```python
from build123d import *

# Parameters (mm, degrees)
SKETCH2_R           = 1.5
BOSS_EXTRUDE1_DEPTH = 2.5
SKETCH3_OUTSIDE_W   = 22.086
SKETCH3_OUTSIDE_H   = 21.158
SKETCH3_OUTSIDE_R   = 3
CUT_EXTRUDE1_DEPTH  = 3.25
CUT_EXTRUDE1_DRAFT  = 60
SKETCH4_OUTSIDE_W   = 22.086
SKETCH4_OUTSIDE_H   = 21.158
SKETCH4_OUTSIDE_R   = 3
CUT_EXTRUDE2_DEPTH  = 3.25
CUT_EXTRUDE2_DRAFT  = -60
CHAMFER1_SIZE       = 0.075


with BuildPart() as part:
    # Sketch2 → Boss-Extrude1 (new body)
    with BuildSketch(Plane(origin=(0, 0, 0), x_dir=(1, 0, 0), z_dir=(0, 1, 0))):
        Polygon((3.464101615, 0), (1.732050808, 3), (-1.732050808, 3), (-3.464101615, 0), (-1.732050808, -3), (1.732050808, -3), align=None)
        with Locations(Location((0, 0, 0), (0, 0, 270))):
            Circle(SKETCH2_R, mode=Mode.SUBTRACT)
    extrude(amount=BOSS_EXTRUDE1_DEPTH)


with BuildPart() as cut_extrude1_tool:
    # Sketch3 outside → Cut-Extrude1 (with draft: the straight prism first)
    with BuildSketch(Plane(origin=(0, 0, 0), x_dir=(1, 0, 0), z_dir=(0, 1, 0))):
        Rectangle(SKETCH3_OUTSIDE_W, SKETCH3_OUTSIDE_H)
        Circle(SKETCH3_OUTSIDE_R, mode=Mode.SUBTRACT)
    extrude(amount=CUT_EXTRUDE1_DEPTH)
    # Cut-Extrude1: the draft: its side faces are tilted about the plane it starts from
    cut_extrude1_sides = [cut_extrude1_tool.faces().sort_by_distance(p)[0] for p in [
        (0, 1.625, 10.579),
        (11.043, 1.625, 0),
        (0, 1.625, -10.579),
        (-11.043, 1.625, 0),
        (-3, 1.625, 0),
    ]]
    draft(cut_extrude1_sides, Plane(origin=(0, 0, 0), x_dir=(1, 0, 0), z_dir=(0, 1, 0)), CUT_EXTRUDE1_DRAFT)


with BuildPart() as part_1:
    add(part.part)

    # Cut-Extrude1: cut by cut_extrude1_tool
    add(cut_extrude1_tool.part, mode=Mode.SUBTRACT)


with BuildPart() as cut_extrude2_tool:
    # Sketch4 outside → Cut-Extrude2 (with draft: the straight prism first)
    with BuildSketch(Plane(origin=(0, 2.5, 0), x_dir=(1, 0, 0), z_dir=(0, 1, 0))):
        Rectangle(SKETCH4_OUTSIDE_W, SKETCH4_OUTSIDE_H)
        Circle(SKETCH4_OUTSIDE_R, mode=Mode.SUBTRACT)
    extrude(amount=-CUT_EXTRUDE2_DEPTH)
    # Cut-Extrude2: the draft: its side faces are tilted about the plane it starts from
    cut_extrude2_sides = [cut_extrude2_tool.faces().sort_by_distance(p)[0] for p in [
        (0, 0.875, 10.579),
        (11.043, 0.875, 0),
        (0, 0.875, -10.579),
        (-11.043, 0.875, 0),
        (-3, 0.875, 0),
    ]]
    draft(cut_extrude2_sides, Plane(origin=(0, 2.5, 0), x_dir=(1, 0, 0), z_dir=(0, 1, 0)), CUT_EXTRUDE2_DRAFT)


with BuildPart() as part_2:
    add(part_1.part)

    # Cut-Extrude2: cut by cut_extrude2_tool
    add(cut_extrude2_tool.part, mode=Mode.SUBTRACT)

    # Chamfer1
    chamfer1_edges = [part_2.edges().sort_by_distance(p)[0] for p in [
        (0, 0, -1.5),
        (0, 2.5, -1.5),
    ]]
    chamfer(chamfer1_edges, length=CHAMFER1_SIZE)


solid = part_2.part
```
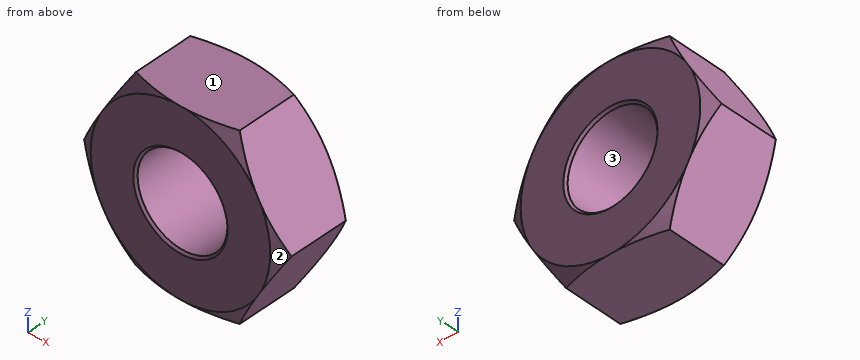
Work out the finished part from the listing and answer in its coordinate system (mm). Face numbers are marked on the shaded views. Give positions to 0.01 mm unless a question says otherwise; leave off trailing zeros. Write each loop counter-clockwise with the first axis right and the second up, starting at its lowest first coordinate (ties: lowest second). Pieces come first, ordered by that corner, then holes. Notation, with made-up numbers: (-12, -14.5) - (-1, -14.5) arc R7 ccw to (-1, -2.5) - close; hole circle Ø4 at (69, -2). An arc over 180 degrees is marked (long way). Use one line per item in the form item = value.
1. Determine the mould class of the marked faces 1, 2 and 3 for opening direction Z: released by +Z, released by -Z, zero draft, split by the parting line, or undercut.
Filled in:
face_1 = released by +Z
face_2 = split by the parting line
face_3 = undercut
2. A cutting plane is placed at A-A (y = 1.5). Write down the section's boundary in (x, z), and give its area (3 significant figures).
Filled in:
outline = (-3.46, 0) - (-1.73, -3) - (1.73, -3) - (3.46, 0) - (1.73, 3) - (-1.73, 3) - close; hole circle Ø3 at (0, 0)
area = 24.1 mm^2
3. Consider L1, parallel to Z at x = -1.25, y = 0.7; L2, parallel to X at y = 1.95, z = -0.25; L3, parallel to Z at x = 0.5, y = 1.4. Determine where each line is inside the solid, lowest interval first.
Filled in:
L1 = -3 to -0.83, 0.83 to 3
L2 = -3.32 to -1.48, 1.48 to 3.32
L3 = -3 to -1.41, 1.41 to 3
